Autodesk Inventor part; units mm, degrees
ref_plane "YZ Plane" through (0, 0, 0) normal (1, 0, 0) x (0, 1, 0)
ref_plane "XZ Plane" through (0, 0, 0) normal (0, 1, 0) x (-1, 0, 0)
ref_plane "XY Plane" through (0, 0, 0) normal (0, 0, 1) x (1, 0, 0)
sketch "Sketch1" plane through (0, 0, 0) normal (0, 0, 1) x (1, 0, 0)
  arc A0 (-2.0086, 7.3505) -> (2.0086, 7.3505) centre (0, 0) ccw
  line L0 (0, 7.62) -> (0, 9.525)
  line L1 (0, 9.525) -> (1.016, 9.525)
  line L2 (0, 9.525) -> (-1.016, 9.525)
  arc A1 (-1.4866, 7.4736) -> (1.4866, 7.4736) centre (0, 0) ccw
  line L3 (-1.4866, 7.4736) -> (-1.8582, 9.342)
  line L4 (-2.916, 7.04) -> (-3.6451, 8.8)
  line L5 (-4.2334, 6.3358) -> (-5.2918, 7.9197)
  line L6 (-5.3882, 5.3882) -> (-6.7352, 6.7352)
  line L7 (-6.3358, 4.2334) -> (-7.9197, 5.2918)
  line L8 (-7.04, 2.916) -> (-8.8, 3.6451)
  line L9 (-7.04, -2.916) -> (-8.8, -3.6451)
  line L10 (-6.3358, -4.2334) -> (-7.9197, -5.2918)
  line L11 (-5.3882, -5.3882) -> (-6.7352, -6.7352)
  line L12 (-4.2334, -6.3358) -> (-5.2918, -7.9197)
  line L13 (-2.916, -7.04) -> (-3.6451, -8.8)
  line L14 (-1.4866, -7.4736) -> (-1.8582, -9.342)
  line L15 (0, -7.62) -> (0, -9.525)
  line L16 (1.4866, -7.4736) -> (1.8582, -9.342)
  line L17 (2.916, -7.04) -> (3.6451, -8.8)
  line L18 (4.2334, -6.3358) -> (5.2918, -7.9197)
  line L19 (5.3882, -5.3882) -> (6.7352, -6.7352)
  line L20 (6.3358, -4.2334) -> (7.9197, -5.2918)
  line L21 (7.04, -2.916) -> (8.8, -3.6451)
  line L22 (7.4736, -1.4866) -> (9.342, -1.8582)
  line L23 (7.62, 0) -> (9.525, 0)
  line L24 (7.4736, 1.4866) -> (9.342, 1.8582)
  line L25 (7.04, 2.916) -> (8.8, 3.6451)
  line L26 (6.3358, 4.2334) -> (7.9197, 5.2918)
  line L27 (5.3882, 5.3882) -> (6.7352, 6.7352)
  line L28 (4.2334, 6.3358) -> (5.2918, 7.9197)
  line L29 (2.916, 7.04) -> (3.6451, 8.8)
  line L30 (1.4866, 7.4736) -> (1.8582, 9.342)
  arc A2 (-1.4866, 7.4736) -> (1.4866, 7.4736) centre (0, 0) ccw
  arc A3 (-1.016, 9.525) -> (-1.6724, 8.4079) centre (-0.1056, 8.2386) ccw
  arc A4 (1.6724, 8.4079) -> (1.016, 9.525) centre (0.1056, 8.2386) ccw
  circle A5 centre (0, 0) radius 7.62
  line L31 (-1.4866, 7.4736) -> (-1.6724, 8.4079)
  line L32 (-1.016, 9.525) -> (1.016, 9.525)
  line L33 (1.6724, 8.4079) -> (1.4866, 7.4736)
  arc A6 (-1.016, 9.525) -> (-1.6724, 8.4079) centre (-0.1056, 8.2386) ccw
  arc A7 (1.6724, 8.4079) -> (1.016, 9.525) centre (0.1056, 8.2386) ccw
  point P0 (-7.4736, 1.4866)
  point P1 (-7.62, 0)
  point P2 (-7.4736, -1.4866)
  dimension "d0" = 15.24
  dimension "d1" = 360
  dimension "d2" = 1.016
  dimension "d3" = 1.016
  dimension "d4" = 1.905
extrude "Extrusion1" add sketch "Sketch1" along normal blind 3.81
pattern_circular "Circular Pattern1" count 8 over 360 about axis through (0, 0, 0) along (0, 0, 1) of "Extrusion1"
sketch "Sketch3" plane through (0, 0, 3.81) normal (0, 0, 1) x (1, 0, 0)
  line L0 (0, 0) -> (0, 1.5)
  line L1 (0, 1.5) -> (2, 1.5)
  line L2 (0, 1.5) -> (-2, 1.5)
  line L3 (0, 0) -> (0.1755, 0)
  line L4 (0, -1.5) -> (2, -1.5)
  line L5 (0, -1.5) -> (-2, -1.5)
  arc A0 (-2, 1.5) -> (-2, -1.5) centre (0, 0) ccw
  arc A1 (2, -1.5) -> (2, 1.5) centre (0, 0) ccw
  dimension "d14" = 1.5
extrude "Extrusion3" cut sketch "Sketch3" against normal up to next
sketch "Sketch4" plane through (0, 0, 3.81) normal (0, 0, 1) x (1, 0, 0)
  circle A0 centre (0, 0) radius 2.5
sketch "Sketch5" plane through (0, 0, 3.81) normal (0, 0, 1) x (1, 0, 0)
  arc A0 (-2, 1.5) -> (-2, -1.5) centre (0, 0) ccw
  line L0 (-2, 1.5) -> (2, 1.5)
  arc A1 (2, -1.5) -> (2, 1.5) centre (0, 0) ccw
  line L1 (2, -1.5) -> (-2, -1.5)
  line L2 (1.4866, 7.4736) -> (1.6724, 8.4079)
  arc A2 (1.6724, 8.4079) -> (1.016, 9.525) centre (0.1056, 8.2386) ccw
  line L3 (1.016, 9.525) -> (-1.016, 9.525)
  arc A3 (-1.016, 9.525) -> (-1.6724, 8.4079) centre (-0.1056, 8.2386) ccw
  line L4 (-1.6724, 8.4079) -> (-1.4866, 7.4736)
  arc A4 (-1.4866, 7.4736) -> (-4.2334, 6.3358) centre (0, 0) ccw
  line L5 (-4.2334, 6.3358) -> (-4.7627, 7.1279)
  arc A5 (-4.7627, 7.1279) -> (-6.0168, 7.4536) centre (-5.7509, 5.9002) ccw
  line L6 (-6.0168, 7.4536) -> (-7.4536, 6.0168)
  arc A6 (-7.4536, 6.0168) -> (-7.1279, 4.7627) centre (-5.9002, 5.7509) ccw
  line L7 (-7.1279, 4.7627) -> (-6.3358, 4.2334)
  arc A7 (-6.3358, 4.2334) -> (-7.4736, 1.4866) centre (0, 0) ccw
  line L8 (-7.4736, 1.4866) -> (-8.4079, 1.6724)
  arc A8 (-8.4079, 1.6724) -> (-9.525, 1.016) centre (-8.2386, 0.1056) ccw
  line L9 (-9.525, 1.016) -> (-9.525, -1.016)
  arc A9 (-9.525, -1.016) -> (-8.4079, -1.6724) centre (-8.2386, -0.1056) ccw
  line L10 (-8.4079, -1.6724) -> (-7.4736, -1.4866)
  arc A10 (-7.4736, -1.4866) -> (-6.3358, -4.2334) centre (0, 0) ccw
  line L11 (-6.3358, -4.2334) -> (-7.1279, -4.7627)
  arc A11 (-7.1279, -4.7627) -> (-7.4536, -6.0168) centre (-5.9002, -5.7509) ccw
  line L12 (-7.4536, -6.0168) -> (-6.0168, -7.4536)
  arc A12 (-6.0168, -7.4536) -> (-4.7627, -7.1279) centre (-5.7509, -5.9002) ccw
  line L13 (-4.7627, -7.1279) -> (-4.2334, -6.3358)
  arc A13 (-4.2334, -6.3358) -> (-1.4866, -7.4736) centre (0, 0) ccw
  line L14 (-1.4866, -7.4736) -> (-1.6724, -8.4079)
  arc A14 (-1.6724, -8.4079) -> (-1.016, -9.525) centre (-0.1056, -8.2386) ccw
  line L15 (-1.016, -9.525) -> (1.016, -9.525)
  arc A15 (1.016, -9.525) -> (1.6724, -8.4079) centre (0.1056, -8.2386) ccw
  line L16 (1.6724, -8.4079) -> (1.4866, -7.4736)
  arc A16 (1.4866, -7.4736) -> (4.2334, -6.3358) centre (0, 0) ccw
  line L17 (4.2334, -6.3358) -> (4.7627, -7.1279)
  arc A17 (4.7627, -7.1279) -> (6.0168, -7.4536) centre (5.7509, -5.9002) ccw
  line L18 (6.0168, -7.4536) -> (7.4536, -6.0168)
  arc A18 (7.4536, -6.0168) -> (7.1279, -4.7627) centre (5.9002, -5.7509) ccw
  line L19 (7.1279, -4.7627) -> (6.3358, -4.2334)
  arc A19 (6.3358, -4.2334) -> (7.4736, -1.4866) centre (0, 0) ccw
  line L20 (7.4736, -1.4866) -> (8.4079, -1.6724)
  arc A20 (8.4079, -1.6724) -> (9.525, -1.016) centre (8.2386, -0.1056) ccw
  line L21 (9.525, -1.016) -> (9.525, 1.016)
  arc A21 (9.525, 1.016) -> (8.4079, 1.6724) centre (8.2386, 0.1056) ccw
  line L22 (8.4079, 1.6724) -> (7.4736, 1.4866)
  arc A22 (7.4736, 1.4866) -> (6.3358, 4.2334) centre (0, 0) ccw
  line L23 (6.3358, 4.2334) -> (7.1279, 4.7627)
  arc A23 (7.1279, 4.7627) -> (7.4536, 6.0168) centre (5.9002, 5.7509) ccw
  line L24 (7.4536, 6.0168) -> (6.0168, 7.4536)
  arc A24 (6.0168, 7.4536) -> (4.7627, 7.1279) centre (5.7509, 5.9002) ccw
  line L25 (4.7627, 7.1279) -> (4.2334, 6.3358)
  arc A25 (4.2334, 6.3358) -> (1.4866, 7.4736) centre (0, 0) ccw
properties part number "8 ul Driver Gear"
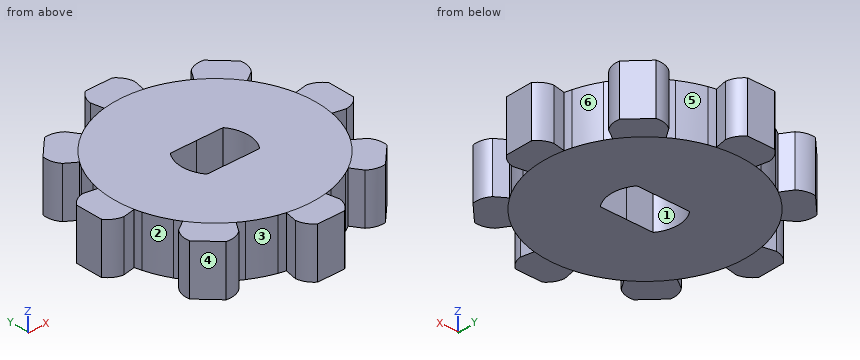
Could you check a few things on this model? Use its own coordinates, in mm. Face numbers are marked on the shaded views. A direction names the side the tool comes from. Coordinates: 2 decimals unless noted, no trailing zeros. Write each loop counter-clockwise with the first axis right and the second up, starting at its lowest first coordinate (ties: lowest second). Pieces come first, ordered by that corner, then holes. Notation, with made-up numbers: M 52.25,85 L 109.25,85 A7 cw 109.25,95 Z; hole C -19.75,-19 d11. An arc over 180 degrees is marked long. Answer as CSV lines item,"result". Start each with the question number.
1) For the marked faces 1, 2 and 3, which set-ups out of +Z, -Z, +X, -X, +Y, -Y let a thin tool reach every point of the face, with its end or its side?
2) For P1, Ø0.6, axis at x = -1.5, z = 1.5, coming from the -Y side, with a flat end and sliding along its axis, tell me the tip position at first contact or that it passes through.
3) I want a section at C-C, the plane x = -5.5. Please give me the cut outline in (y, z), and give its area (3 significant figures).
4) Please list where these lines run through material, in increasing order: line 1 (X direction, y = 6.75, z = 3.55); line 2 (Y direction, x = -1, z = 2.5) (3 decimals); line 3 (X direction, y = 7, z = 1.4). Write a range as from..to.
5) I want a section at A-A, the plane x = 0.75. Please give me the cut outline in (y, z) (3 decimals), and give its area (3 significant figures).
6) I want a section at B-B, the plane y = 4. Please give me the cut outline in (x, z).
7) We'd pull the mould along X, two halves only. Please class the marked faces 4, 5 and 6: +X half, -X half, draft (parallel to the pull), parting line (faces both ways), or undercut.
Data:
1,face 1,"+Z, -Z"
1,face 2,"+Z, -Z, -X"
1,face 3,"+Z, -Z, -Y"
2,P1,"stops at y = -9.37"
3,outline,"M -7.46,0 L 7.46,0 L 7.46,3.81 L -7.46,3.81 Z"
3,area,"56.8 mm^2"
4,line 1,"x = -6.72..-4.51, -3.54..3.54, 4.51..6.72"
4,line 2,"y = -9.525..-1.5, 1.5..9.525"
4,line 3,"x = -6.47..-4.68, -3.01..3.01, 4.68..6.47"
5,outline,"M -9.525,0 L -1.5,0 L -1.5,3.81 L -9.525,3.81 Z; M 1.5,0 L 9.525,0 L 9.525,3.81 L 1.5,3.81 Z"
5,area,"61.2 mm^2"
6,outline,"M -6.49,0 L 6.49,0 L 6.49,3.81 L -6.49,3.81 Z"
7,face 4,"-X half"
7,face 5,"undercut"
7,face 6,"+X half"
